Here's how the part is built. I have some questions about the finished solid (model axes, mm). Round coordinates to 2 decimals unless told otherwise and drop trailing zeros. Write each loop counter-clockwise with the first axis right and the second up, starting at its lowest first coordinate (ties: lowest second). Pieces come first, ordered by that corner, then holes. Notation, with made-up numbers: (52.5, -34.75) -> (92.5, -34.75) arc R23 cw to (92.5, -11.75) -> close; hole circle Ø8 at (-16, 5). An arc over 180 degrees is marked (long way). Put each result on its own line as item: value. Start each with the question number.
1) I want a section at A-A, the plane x = -17.5. List the corners of the cut face in (y, z) for me, then the cut area to 3 significant figures.
2) I want a section at C-C, the plane x = 1.5. List the corners of the cut face in (y, z) for me.
3) Will this pin go through, and if not, where does the flat tip stop? P1, Ø1.5, axis at x = -17.5, y = -2, coming from the -Z side.
4) I want a section at B-B, the plane x = 24. List the corners of the cut face in (y, z) for me.
5) If I drill on line 1 along Z through (x, y) = (-18, -1.4); line 2 along X through (y, z) = (-1.9, 35.75); line 3 along Z through (x, y) = (-11, -1.45), over which ranges is the centre line in solid material (lowest first)? Write a range as [from, to].
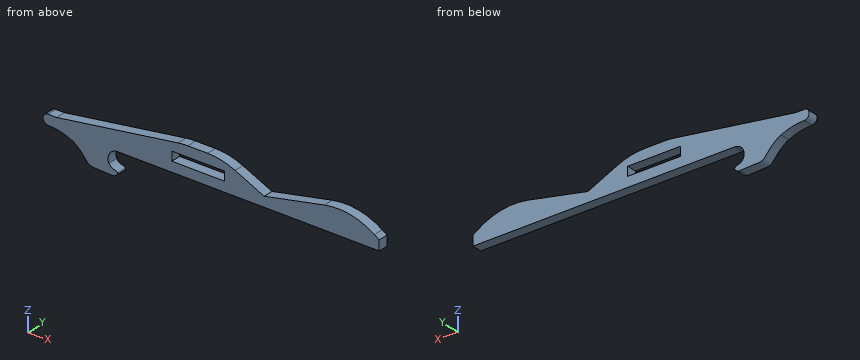
from build123d import *

# Parameters (mm, degrees)
F1_DEPTH = 3


with BuildPart() as f1:
    # F0 (on Front) → F1 (new body)
    with BuildSketch(Plane.XZ):
        with BuildLine():
            Line((-62.2174302257, 34.0792866244), (-62.2174302257, 37.0792866244))
            ThreePointArc((-62.2174302257, 37.0792866244), (-63.7174302257, 35.5792866244), (-62.2174302257, 34.0792866244))
        make_face()
        with BuildLine():
            ThreePointArc((-43.8397750258, 30.0628747791), (-43.6141613241, 32.781176986), (-41.2152074277, 34.0792866244))
            Line((-41.2152074277, 34.0792866244), (-41.2691645324, 34.0792866244))
            Line((-41.2691645324, 34.0792866244), (-54.0572144091, 34.0792866244))
            Line((-54.0572144091, 34.0792866244), (-62.2174302257, 34.0792866244))
            ThreePointArc((-62.2174302257, 34.0792866244), (-58.6487465395, 33.6917698382), (-55.2464202046, 32.5472839177))
            add(Edge.make_bspline(
                [(-42.7791178226, 27.0931944251), (-49.7212063405, 27.3062232623), (-49.3171741888, 27.0847515739), (-53.5192862103, 31.93581339), (-55.2464202046, 32.5472839177)],
                knots=[0, 0, 0, 0, 0.5316142491, 1, 1, 1, 1], degree=3))
            add(Edge.make_bspline(
                [(-43.8397750258, 30.0628747791), (-42.9603002793, 28.648200624), (-40.4412665904, 29.1570281848), (-41.5067049695, 27.1511407727), (-42.7791178226, 27.0931944251)],
                knots=[0, 0, 0, 0, 0.5503485868, 1, 1, 1, 1], degree=3))
        make_face()
        with BuildLine():
            Line((-8.9188218117, 37.0792866244), (3.0751132872, 37.0792866244))
            Line((3.0751132872, 37.0792866244), (-5.7411652831, 41.0951580407))
            ThreePointArc((-5.7411652831, 41.0951580407), (-9.7899424344, 42.4394313305), (-14.0317167887, 42.894423008))
            Line((-14.0317167887, 42.894423008), (-19.9778148896, 42.894423008))
            ThreePointArc((-19.9778148896, 42.894423008), (-21.4905036729, 42.837135277), (-22.9945266053, 42.6656002725))
            Line((-22.9945266053, 42.6656002725), (-59.6065756835, 37.0792866244))
            Line((-59.6065756835, 37.0792866244), (-24.8117092997, 37.0792866244))
            Line((-24.8117092997, 37.0792866244), (-24.8117092997, 39.829544723))
            Line((-24.8117092997, 39.829544723), (-8.9188218117, 39.829544723))
            Line((-8.9188218117, 39.829544723), (-8.9188218117, 37.0792866244))
        make_face()
        Polygon((37.7825697743, 34.0792866244), (37.7825697743, 37.0792866244), (3.0751132872, 37.0792866244), (-8.9188218117, 37.0792866244), (-24.8117092997, 37.0792866244), (-59.6065756835, 37.0792866244), (-62.2174302257, 37.0792866244), (-62.2174302257, 34.0792866244), (-54.0572144091, 34.0792866244), (-41.2691645324, 34.0792866244), (-41.2152074277, 34.0792866244), align=None)
        with BuildLine():
            Line((3.0751132872, 37.0792866244), (37.7825697743, 37.0792866244))
            Line((37.7825697743, 37.0792866244), (36.3480403802, 38.0231242511))
            ThreePointArc((36.3480403802, 38.0231242511), (29.0861642169, 40.964055469), (21.251728148, 40.889669157))
            Line((21.251728148, 40.889669157), (3.0751132872, 37.0792866244))
        make_face()
    extrude(amount=F1_DEPTH)


solid = f1.part
Findings:
1. outline: (-3, 34.08) -> (0, 34.08) -> (0, 37.08) -> (-3, 37.08) -> close; (-3, 39.83) -> (0, 39.83) -> (0, 42.89) -> (-3, 42.89) -> close
1. area: 18.2 mm2
2. outline: (-3, 34.08) -> (0, 34.08) -> (0, 37.8) -> (-3, 37.8) -> close
3. P1: stops at z = 34.08
4. outline: (-3, 34.08) -> (0, 34.08) -> (0, 41.27) -> (-3, 41.27) -> close
5. line 1: z = [34.08, 37.08], [39.83, 42.89]
5. line 2: x = [-63.71, 37.78]
5. line 3: z = [34.08, 37.08], [39.83, 42.66]
